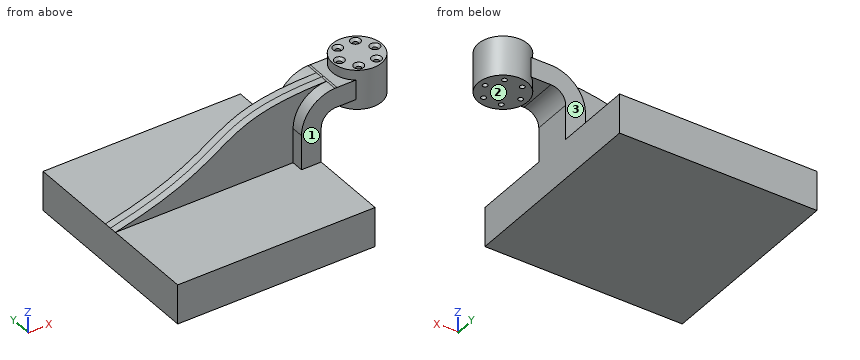
from build123d import *

# Parameters (mm, degrees)
F1_DEPTH        = 100
F0_W            = 25
F0_H            = 20
F2_DEPTH        = 20
F3_DEPTH        = 7.5
F6_D            = 5
F6_CSINK_D      = 10
F6_CSINK_ANGLE  = 90
F6_COPIES_COUNT = 6


# Not quite as in the source:
# - a pattern or mirror of a feature is missing from the dataset's text; its kind, count and spacing are read off the source's solid


with BuildPart() as f1:
    # F0 (on Front) → F1 (new body, symmetric)
    with BuildSketch(Plane.XZ):
        Polygon((-100, -20), (100, -20), (100, 20), (80, 20), (-100, 20), align=None)
    extrude(amount=F1_DEPTH, both=True)

    # F0 (on Front) → F2 (join, symmetric)
    with BuildSketch(Plane.XZ):
        with BuildLine():
            Line((80, 20), (100, 20))
            Line((100, 20), (100, 55))
            ThreePointArc((100, 55), (104.3933982822, 65.6066017178), (115, 70))
            Line((115, 70), (125, 70))
            Line((125, 70), (125, 90))
            Line((125, 90), (116.0234387074, 90))
            add(Edge.make_bspline(
                [(113.8611942755, 89.9814682585), (114.576343668, 89.9888687938), (115.2970695321, 89.9950487976), (116.0234387074, 90)],
                knots=[228.983844188, 228.983844188, 228.983844188, 228.983844188, 230.3162896959, 230.3162896959, 230.3162896959, 230.3162896959], degree=3))
            ThreePointArc((113.8611942755, 89.9814682585), (89.8518569238, 79.3427792132), (80, 55))
            Line((80, 55), (80, 20))
        make_face()
        with Locations((137.5, 80)):
            Rectangle(F0_W, F0_H)
    extrude(amount=F2_DEPTH, both=True)

    # F0 (on Front) → F3 (join, symmetric)
    with BuildSketch(Plane.XZ):
        with BuildLine():
            add(Edge.make_bspline(
                [(-100, 20), (32.7521878521, 51.3916469178), (-9.0388838859, 88.7096691401), (113.8611942755, 89.9814682585)],
                knots=[0, 0, 0, 0, 228.983844188, 228.983844188, 228.983844188, 228.983844188], degree=3))
            Line((-100, 20), (80, 20))
            Line((80, 20), (80, 55))
            ThreePointArc((80, 55), (89.8518569238, 79.3427792132), (113.8611942755, 89.9814682585))
        make_face()
    extrude(amount=F3_DEPTH, both=True)

    # F0 (on Front) → F4 (revolve)
    with BuildSketch(Plane.XZ):
        Polygon((150, 90), (150, 70), (150, 60), (175, 60), (175, 100), (150, 100), align=None)
    revolve(axis=Axis((150, 0, 80), (0, 0, 1)))

    # F6 (through all)
    with Locations(Plane.XY.offset(100)):
        with Locations((168, 0)):
            f6 = CounterSinkHole(F6_D / 2, F6_CSINK_D / 2, counter_sink_angle=F6_CSINK_ANGLE)

    # F6_copies: F6 ×6 about axis
    f6_copies_axis = Axis((150, 0, 0), (0, 0, 1))
    for i in range(1, F6_COPIES_COUNT):
        add(f6.rotate(f6_copies_axis, i * 360 / F6_COPIES_COUNT), mode=Mode.SUBTRACT)


solid = f1.part
Input: part model. Units: mm. Frame: model coordinates. Face numbers are marked on the shaded views. A direction names the side the tool comes from. Give positions to 0.01 mm unless a question says otherwise; leave off trailing zeros. Order: outer loops, then holes, each group sorted by start corner. A loop starts at its lowest first (then second) coordinate and runs counter-clockwise, first axis right, second up. Notation, with made-up numbers: (31.25, -4) - (54.25, -4) arc R28 cw to (54.25, 14) - close; hole circle Ø6 at (52.5, 55.5). An arc over 180 degrees is marked (long way). Answer as a JSON object with one key per item and string values. Group by question number.
Q1. Set-up query: the marked faces 1, 2 and 3. Return all of +Z, -Z, +X, -X, +Y, -Y with unobstructed straight access to the full face (end or side cutting, diameter ignored); none if empty.
Q2. First-contact query: pin 1 Ø15 at (x, y) = (146, -11.5) entering from -Z; pin 2 Ø4 at (y, z) = (13.5, 45) entering from -X; pin 3 Ø6 at (x, z) = (76.5, 84.5) entering from -Y. Flat tips, straight axial feed; report the tip coordinate or a pass-through.
Q3. Cut plane A-A, the plane z = 5. Output: boundary loops of the cut face in (x, y).
Q4. Cut plane B-B, the plane y = 66. Output: boundary loops of the cut face in (x, z), then the cut area to 3 significant figures.
Q5. Cut plane C-C, the plane z = 78.5. Count the separate pieces of the cut face and the enclosed holes in it, then the cut area to 3 significant figures.
Q6. Line query: probe 1 along Y at (x, z) = (132, 72); probe 2 along Y at (x, z) = (159, 71.5); probe 3 along Z at (x, y) = (-54.5, -60). Output: solid intervals per line, ascending.
Results:
{
 "1": {"face 1": "+Z, -X, -Y", "face 2": "-Z, +X, +Y, -Y", "face 3": "+Z, -X, +Y"},
 "2": {"pin 1": "z = 60", "pin 2": "x = 80", "pin 3": "y = -7.5"},
 "3": {"outline": "(-100, -100) - (100, -100) - (100, 100) - (-100, 100) - close"},
 "4": {"outline": "(-100, -20) - (100, -20) - (100, 20) - (-100, 20) - close", "area": "8,000 mm^2"},
 "5": {"separate pieces": "1", "enclosed holes": "6", "area": "4,230 mm^2"},
 "6": {"probe 1": "-20 to -2.5, 2.5 to 20", "probe 2": "-23.32 to -18.09, -13.09 to 13.09, 18.09 to 23.32", "probe 3": "-20 to 20"}
}
